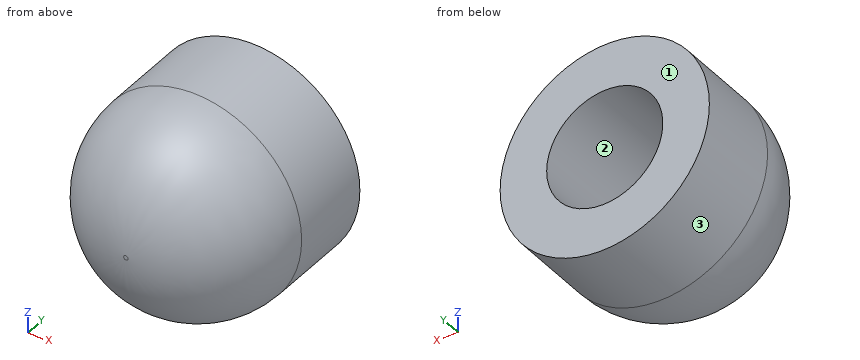
from build123d import *

# Parameters (mm, degrees)
F0_R     = 285.475239
F1_DEPTH = 508
F2_T     = -127
F3_R     = 279.4


with BuildPart() as f1:
    # F0 (on Front) → F1 (new body)
    with BuildSketch(Plane.XZ):
        Circle(F0_R)
    extrude(amount=F1_DEPTH)

    # F2
    f2_openings = [f1.faces().sort_by_distance(p)[0] for p in [
        (0, 0, 0),
    ]]
    offset(amount=F2_T, openings=f2_openings)

    # F3
    f3_edges = [f1.edges().sort_by_distance(p)[0] for p in [
        (-285.475239, -508, 0),
    ]]
    fillet(f3_edges, radius=F3_R)


solid = f1.part
Work out the finished part from the listing and answer in its coordinate system (mm). Face numbers are marked on the shaded views. Give positions to 0.01 mm unless a question says otherwise; leave off trailing zeros. Order: outer loops, then holes, each group sorted by start corner. A loop starts at its lowest first (then second) coordinate and runs counter-clockwise, first axis right, second up. Notation, with made-up numbers: (77.25, -17) -> (133.25, -17) arc R9 cw to (133.25, -2) -> close; hole circle Ø11 at (-8, -18.75). An arc over 180 degrees is marked (long way). Answer as a JSON object with one key per item and string values. Group by question number.
1. Consider line 1 along Z through (x, y) = (0, -141.5); line 2 along X through (y, z) = (-202, -21); line 3 along X through (y, z) = (-341, -34). Determine where each line is inside the solid, lowest interval first. Write a range as [from, to].
2. The mould has two halves that part along X. Classify the marked faces 1, 2 and 3: released by +X, released by -X, zero draft, split by the parting line, or undercut.
3. Flat-ended cylindrical pins translate along their axes: pin 1 Ø3 at (x, z) = (125, -73) entering from -Y; pin 2 Ø1 at (x, y) = (-168, -105.5) entering from -Z; pin 3 Ø4 at (x, y) = (-170.5, -301.5) entering from -Z. Find the tip coordinate at first contact, or state that the pin passes through.
4. Section A-A on y = -200 is taken. Determine the outline of the cut face in (x, z).
Result sheet:
{
 "1": {"line 1": "z = [-285.48, -158.48], [158.48, 285.48]", "line 2": "x = [-284.7, -157.08], [157.08, 284.7]", "line 3": "x = [-259.65, -154.79], [154.79, 259.65]"},
 "2": {"face 1": "zero draft", "face 2": "undercut", "face 3": "split by the parting line"},
 "3": {"pin 1": "stops at y = -472.01", "pin 2": "stops at z = -231.17", "pin 3": "stops at z = -218.48"},
 "4": {"outline": "circle Ø570.95 at (0, 0); hole circle Ø316.95 at (0, 0)"}
}
